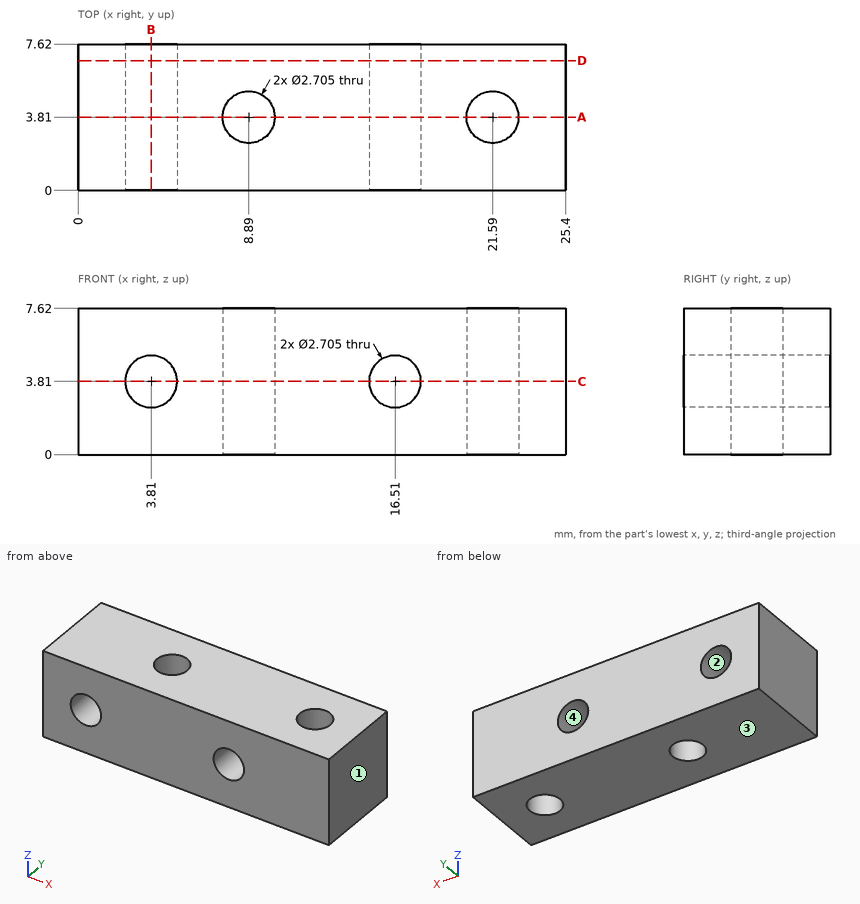
For this review, use the dimensioned drawing (mm, ordinates from the lowest corner) and the shaded views. Coordinates: 2 decimals unless noted, no trailing zeros. Write each loop counter-clockwise with the first axis right and the second up, starting at its lowest first coordinate (ties: lowest second). Pieces come first, ordered by that corner, then holes. Notation, with made-up numbers: (-14.75, 77.25) - (40.25, 77.25) arc R12 cw to (40.25, 98.25) - close; hole circle Ø11 at (2.25, 34). An arc over 180 degrees is marked (long way). Answer as a JSON object with one key per item and string values. Group by question number.
1. To check wall thickness, follow probe 1 along Z at (x, y) = (3.81, 5.5); probe 2 along X at (y, z) = (3, 2.25). State the ranges of each line that lie inside material, in increasing order.
2. Mouldability with a two-part tool opening along Z and no side actions: class the marked faces 1, 2, 3 and 4 as pulls with the +Z half, pulls with the -Z half, needs draft (parallel to the pull), parting line crosses it, or undercut.
3. Add section C-C (z = 3.81). Give the boundary of the cut face in (x, y) (1 decimal).
4. Add section A-A (y = 3.81). Give the boundary of the cut face in (x, z) (1 decimal).
5. Add section D-D (y = 6.75). Give the boundary of the cut face in (x, z) (1 decimal), plus the area to 3 significant figures.
6. Add section B-B (x = 3.81). Give the boundary of the cut face in (y, z).
Findings:
{
 "1": {"probe 1": "0 to 2.46, 5.16 to 7.62", "probe 2": "0 to 7.81, 9.97 to 20.51, 22.67 to 25.4"},
 "2": {"face 1": "needs draft", "face 2": "undercut", "face 3": "pulls with the -Z half", "face 4": "undercut"},
 "3": {"outline": "(0, 0) - (2.5, 0) - (2.5, 7.6) - (0, 7.6) - close; (5.2, 0) - (15.2, 0) - (15.2, 7.6) - (5.2, 7.6) - close; (17.9, 0) - (25.4, 0) - (25.4, 7.6) - (17.9, 7.6) - close; hole circle Ø2.7 at (8.9, 3.8); hole circle Ø2.7 at (21.6, 3.8)"},
 "4": {"outline": "(0, 0) - (7.5, 0) - (7.5, 7.6) - (0, 7.6) - close; (10.2, 0) - (20.2, 0) - (20.2, 7.6) - (10.2, 7.6) - close; (22.9, 0) - (25.4, 0) - (25.4, 7.6) - (22.9, 7.6) - close; hole circle Ø2.7 at (3.8, 3.8); hole circle Ø2.7 at (16.5, 3.8)"},
 "5": {"outline": "(0, 0) - (25.4, 0) - (25.4, 7.6) - (0, 7.6) - close; hole circle Ø2.7 at (3.8, 3.8); hole circle Ø2.7 at (16.5, 3.8)", "area": "182 mm²"},
 "6": {"outline": "(0, 0) - (7.62, 0) - (7.62, 2.46) - (0, 2.46) - close; (0, 5.16) - (7.62, 5.16) - (7.62, 7.62) - (0, 7.62) - close"}
}
